```python
from build123d import *

# Parameters (mm, degrees)
SKETCH1_W           = 90
SKETCH1_H           = 16
BOSS_EXTRUDE1_DEPTH = 5
SKETCH2_W           = 90
SKETCH2_H           = 3
BOSS_EXTRUDE2_DEPTH = 3
SKETCH3_R           = 2
CUT_EXTRUDE2_DEPTH  = 5
SKETCH4_W           = 90
SKETCH4_H           = 16
SKETCH4_R           = 2
BOSS_EXTRUDE3_DEPTH = 5
SKETCH5_W           = 90
SKETCH5_H           = 3
BOSS_EXTRUDE4_DEPTH = 3
BOSS_EXTRUDE5_DEPTH = 5
SKETCH7_W           = 3
SKETCH7_H           = 75
BOSS_EXTRUDE6_DEPTH = 3
SKETCH8_R           = 2
CUT_EXTRUDE5_DEPTH  = 5
SKETCH9_R           = 2
CUT_EXTRUDE6_DEPTH  = 5
FILLET1_R           = 5
SKETCH10_R          = 4
CUT_EXTRUDE7_DEPTH  = 2
SKETCH11_R          = 4
CUT_EXTRUDE8_DEPTH  = 2


with BuildPart() as part:
    # Sketch1 → Boss-Extrude1 (new body)
    with BuildSketch(Plane(origin=(0, 0, 0), x_dir=(1, 0, 0), z_dir=(0, 1, 0))):
        with Locations((-6.794417438, 1.807142857)):
            Rectangle(SKETCH1_W, SKETCH1_H)
    extrude(amount=BOSS_EXTRUDE1_DEPTH)

    # Sketch2 → Boss-Extrude2 (add)
    with BuildSketch(Plane(origin=(0, 5, 0), x_dir=(1, 0, 0), z_dir=(0, 1, 0))):
        with Locations((-6.794417438, 8.307142857)):
            Rectangle(SKETCH2_W, SKETCH2_H)
        with Locations((-6.794417438, -4.692857143)):
            Rectangle(SKETCH2_W, SKETCH2_H)
    extrude(amount=BOSS_EXTRUDE2_DEPTH)

    # Sketch3 → Cut-Extrude2 (cut)
    with BuildSketch(Plane.XZ):
        with Locations(Location((20.205582562, -1.807142857, 0), (0, 0, 270))):
            Circle(SKETCH3_R)
        with Locations(Location((-22.794417438, -1.807142857, 0), (0, 0, 270))):
            Circle(SKETCH3_R)
    extrude(amount=-CUT_EXTRUDE2_DEPTH, mode=Mode.SUBTRACT)



with BuildPart() as body_2:
    # Sketch4 → Boss-Extrude3 (new body)
    with BuildSketch(Plane.XZ):
        with Locations((-6.794417438, -92.807142857)):
            Rectangle(SKETCH4_W, SKETCH4_H)
        with Locations(Location((20.205582562, -92.807142857, 0), (0, 0, 270))):
            Circle(SKETCH4_R, mode=Mode.SUBTRACT)
        with Locations(Location((-22.794417438, -92.807142857, 0), (0, 0, 270))):
            Circle(SKETCH4_R, mode=Mode.SUBTRACT)
    extrude(amount=-BOSS_EXTRUDE3_DEPTH)

    # Sketch5 → Boss-Extrude4 (add)
    with BuildSketch(Plane(origin=(0, 5, 0), x_dir=(1, 0, 0), z_dir=(0, 1, 0))):
        with Locations((-6.794417438, 99.307142857)):
            Rectangle(SKETCH5_W, SKETCH5_H)
        with Locations((-6.794417438, 86.307142857)):
            Rectangle(SKETCH5_W, SKETCH5_H)
    extrude(amount=BOSS_EXTRUDE4_DEPTH)


with BuildPart() as part_1:
    add(part.part)

    add(body_2.part)  # Boss-Extrude5 merges body 2
    # Sketch6 → Boss-Extrude5 (add)
    with BuildSketch(Plane.XZ):
        Polygon((-6.794417438, -84.807142857), (1.205582562, -84.807142857), (1.205582562, -9.807142857), (-14.794417438, -9.807142857), (-14.794417438, -84.807142857), align=None)
    extrude(amount=-BOSS_EXTRUDE5_DEPTH)

    # Sketch7 → Boss-Extrude6 (add)
    with BuildSketch(Plane(origin=(0, 5, 0), x_dir=(1, 0, 0), z_dir=(0, 1, 0))):
        with Locations((-0.294417438, 47.307142857)):
            Rectangle(SKETCH7_W, SKETCH7_H)
        with Locations((-13.294417438, 47.307142857)):
            Rectangle(SKETCH7_W, SKETCH7_H)
    extrude(amount=BOSS_EXTRUDE6_DEPTH)

    # Sketch8 → Cut-Extrude5 (cut)
    with BuildSketch(Plane(origin=(0, 5, 0), x_dir=(1, 0, 0), z_dir=(0, 1, 0))):
        with Locations(Location((-46.794417438, 92.807142857, 0), (0, 0, 270))):
            Circle(SKETCH8_R)
        with Locations(Location((-34.794417438, 92.807142857, 0), (0, 0, 270))):
            Circle(SKETCH8_R)
        with Locations(Location((29.205582562, 92.807142857, 0), (0, 0, 270))):
            Circle(SKETCH8_R)
        with Locations(Location((9.455582562, 92.807142857, 0), (0, 0, 270))):
            Circle(SKETCH8_R)
        with Locations(Location((-1.294417438, 92.807142857, 0), (0, 0, 270))):
            Circle(SKETCH8_R)
        with Locations(Location((-12.044417438, 92.807142857, 0), (0, 0, 270))):
            Circle(SKETCH8_R)
        with Locations(Location((-1.294417438, 1.807142857, 0), (0, 0, 270))):
            Circle(SKETCH8_R)
        with Locations(Location((-12.044417438, 1.807142857, 0), (0, 0, 270))):
            Circle(SKETCH8_R)
        with Locations(Location((9.455582562, 1.807142857, 0), (0, 0, 270))):
            Circle(SKETCH8_R)
        with Locations(Location((-34.794417438, 1.807142857, 0), (0, 0, 270))):
            Circle(SKETCH8_R)
        with Locations(Location((29.205582562, 1.807142857, 0), (0, 0, 270))):
            Circle(SKETCH8_R)
        with Locations(Location((-46.794417438, 1.807142857, 0), (0, 0, 270))):
            Circle(SKETCH8_R)
    extrude(amount=-CUT_EXTRUDE5_DEPTH, mode=Mode.SUBTRACT)

    # Sketch9 → Cut-Extrude6 (cut)
    with BuildSketch(Plane(origin=(0, 5, 0), x_dir=(1, 0, 0), z_dir=(0, 1, 0))):
        with Locations(Location((-6.794417438, 47.307142857, 0), (0, 0, 270))):
            Circle(SKETCH9_R)
        with Locations(Location((-6.794417438, 57.307142857, 0), (0, 0, 270))):
            Circle(SKETCH9_R)
        with Locations(Location((-6.794417438, 67.307142857, 0), (0, 0, 270))):
            Circle(SKETCH9_R)
        with Locations(Location((-6.794417438, 77.307142857, 0), (0, 0, 270))):
            Circle(SKETCH9_R)
        with Locations(Location((-6.794417438, 37.307142857, 0), (0, 0, 270))):
            Circle(SKETCH9_R)
        with Locations(Location((-6.794417438, 27.307142857, 0), (0, 0, 270))):
            Circle(SKETCH9_R)
        with Locations(Location((-6.794417438, 17.307142857, 0), (0, 0, 270))):
            Circle(SKETCH9_R)
    extrude(amount=-CUT_EXTRUDE6_DEPTH, mode=Mode.SUBTRACT)

    # Fillet1
    fillet1_edges = [part_1.edges().sort_by_distance(p)[0] for p in [
        (-14.794417438, 4, -84.807142857),
        (-14.794417438, 4, -9.807142857),
        (1.205582562, 4, -9.807142857),
        (1.205582562, 4, -84.807142857),
    ]]
    fillet(fillet1_edges, radius=FILLET1_R)

    # Sketch10 → Cut-Extrude7 (cut)
    with BuildSketch(Plane.XZ):
        with Locations(Location((20.205582562, -1.807142857, 0), (0, 0, 270))):
            Circle(SKETCH10_R)
        with Locations(Location((-22.794417438, -1.807142857, 0), (0, 0, 270))):
            Circle(SKETCH10_R)
        with Locations(Location((20.205582562, -92.807142857, 0), (0, 0, 270))):
            Circle(SKETCH10_R)
        with Locations(Location((-22.794417438, -92.807142857, 0), (0, 0, 270))):
            Circle(SKETCH10_R)
    extrude(amount=-CUT_EXTRUDE7_DEPTH, mode=Mode.SUBTRACT)

    # Sketch11 → Cut-Extrude8 (cut)
    with BuildSketch(Plane.XZ):
        with Locations(Location((-46.794417438, -1.807142857, 0), (0, 0, 270))):
            Circle(SKETCH11_R)
        with Locations(Location((-46.794417438, -92.807142857, 0), (0, 0, 270))):
            Circle(SKETCH11_R)
    extrude(amount=-CUT_EXTRUDE8_DEPTH, mode=Mode.SUBTRACT)


solid = part_1.part
```
Geometry: final body of the model. Coordinates: model frame, mm. A direction names the side the tool comes from. Round coordinates to 2 decimals unless told otherwise and drop trailing zeros. Write each loop counter-clockwise with the first axis right and the second up, starting at its lowest first coordinate (ties: lowest second). Pieces come first, ordered by that corner, then holes. Notation, with made-up numbers: M 11,36.5 L 26,36.5 A26 cw 26,71.5 Z; hole C -7,-6 d9. An arc over 180 degrees is marked long. Answer in a Markdown table with one row per item. Add a question column.
(1) Ray query, L1, parallel to Z at x = 30.5, y = 6.75; L2, parallel to Z at x = -1, y = 5.25; L3, parallel to Z at x = 10, y = 4. Return the intervals inside material, ascending.
(2) Cut plane A-A, the plane y = 6.75. Return the cut outline in (x, z).
(3) Cut plane C-C, the plane z = -43.5. Return the cut outline in (x, y).
(4) Cut plane D-D, the plane z = -17. Return the cut outline in (x, y).
(5) Draft query along X for faces 5 (the face through (-7, 4, 6.193)), 6 (the face through (20.38, 0.99, -88.81)), 7 (the face through (-46.62, 0.99, -88.81)), 8 (the face through (2.63, 3.94, -11.31)). Return one class per face: pulls with the +X half, pulls with the -X half, needs draft (parallel to the pull), parting line crosses it, or undercut.
(6) Contact query for flat-ended pins moving along their axis: pin 1 (3 mm diameter, centred on x = -9, z = -51, fed in from +Y); pin 2 (3.5 mm diameter, centred on x = -1.29, z = -1.81, fed in from +Y); pin 3 (7 mm diameter, centred on x = -22.79, z = -92.81, fed in from -Y). Output: stop coordinate, or through.
(7) Cut plane B-B, the plane x = -38. Return the cut outline in (y, z).
(8) Reachability of faces 1 (the face through (-16.22, 3.94, -11.31)), 2 (the face through (-7, 6, -84.807)), 3 (the face through (38.206, 3, -93)), 4 (the face through (-7, 6, -6.807)) from +Z, -Z, +X, -X, +Y, -Y: full face, straight path, thin tool, end or side. Return the list, or none.
Established:
| question | item | result |
|---|---|---|
| 1 | L1 | -100.81 to -97.81, -87.81 to -84.81, -9.81 to -6.81, 3.19 to 6.19 |
| 1 | L2 | -100.81 to -97.81, -87.81 to -6.81, 3.19 to 6.19 |
| 1 | L3 | -100.81 to -94.73, -90.88 to -84.81, -9.81 to -3.73, 0.12 to 6.19 |
| 2 | outline | M -51.79,-100.81 L 38.21,-100.81 L 38.21,-97.81 L -51.79,-97.81 Z; M -51.79,-87.81 L 38.21,-87.81 L 38.21,-84.81 L 6.21,-84.81 A5 cw 1.21,-79.81 L 1.21,-14.81 A5 cw 6.21,-9.81 L 38.21,-9.81 L 38.21,-6.81 L -51.79,-6.81 L -51.79,-9.81 L -19.79,-9.81 A5 cw -14.79,-14.81 L -14.79,-79.81 A5 cw -19.79,-84.81 L -51.79,-84.81 Z; M -51.79,3.19 L 38.21,3.19 L 38.21,6.19 L -51.79,6.19 Z; hole M -11.79,-84.81 L -1.79,-84.81 L -1.79,-9.81 L -11.79,-9.81 Z |
| 3 | outline | M -14.79,0 L 1.21,0 L 1.21,8 L -1.79,8 L -1.79,5 L -11.79,5 L -11.79,8 L -14.79,8 Z |
| 4 | outline | M -14.79,0 L -8.77,0 L -8.77,5 L -11.79,5 L -11.79,8 L -14.79,8 Z; M -4.82,0 L 1.21,0 L 1.21,8 L -1.79,8 L -1.79,5 L -4.82,5 Z |
| 5 | face 5 | needs draft |
| 5 | face 6 | undercut |
| 5 | face 7 | undercut |
| 5 | face 8 | pulls with the +X half |
| 6 | pin 1 | y = 5 |
| 6 | pin 2 | through |
| 6 | pin 3 | y = 2 |
| 7 | outline | M 0,-100.81 L 8,-100.81 L 8,-97.81 L 5,-97.81 L 5,-87.81 L 8,-87.81 L 8,-84.81 L 0,-84.81 Z; M 0,-9.81 L 8,-9.81 L 8,-6.81 L 5,-6.81 L 5,3.19 L 8,3.19 L 8,6.19 L 0,6.19 Z |
| 8 | face 1 | -X, +Y, -Y |
| 8 | face 2 | +Y |
| 8 | face 3 | +Z, -Z, +X, +Y, -Y |
| 8 | face 4 | +X, -X, +Y |
